Build history of the part. All positions in model axes, mm. Face numbers are marked on the shaded views. A direction names the side the tool comes from. Give positions to 0.01 mm unless a question says otherwise; leave off trailing zeros. Write each loop counter-clockwise with the first axis right and the second up, starting at its lowest first coordinate (ties: lowest second). Pieces come first, ordered by that corner, then holes. Notation, with made-up numbers: (50.5, -13) -> (104.5, -13) arc R11 ccw to (104.5, -5) -> close; hole circle Ø11 at (-16, -21). An arc over 180 degrees is marked (long way). Write item = value, one per line. Start each with the question number.
Q1. Saw through at A-A, the plane y = 0. List the corners of the cut face in (x, z).
Q2. Mould opens along Y. For the marked faces 4, 5 and 6 say: pulls with the +Y half, pulls with the -Y half, needs draft (parallel to the pull), parting line crosses it, or undercut.
Q3. Saw through at D-D, the plane y = -13.5. List the corners of the cut face in (x, z), then the cut area to 3 significant figures.
Q4. Tool access for the marked faces 1, 2 and 3: list every direction of +Z, -Z, +X, -X, +Y, -Y with a clear straight run to the whole face (end or side of a thin tool).
Q5. Drop flat-ended pins along their axis: P1, Ø4, axis at y = -4, z = 3.5, coming from the +X side; P2, Ø21, axis at x = 0, y = 0, coming from the +Z side; P3, Ø3, axis at x = 14.5, z = 3, coming from the +Y side. Give the stop position or say it passes through.
Q6. Wall check: line 1 (Y direction, x = 0, z = 3.5); line 2 (Y direction, x = 0, z = -0.5); line 3 (Z direction, x = -12, y = -19). Give the ranges that are in metal, low to high.
Q7. Saw through at C-C, the plane z = 4. List the corners of the cut face in (x, y), then the cut area to 3 significant figures.
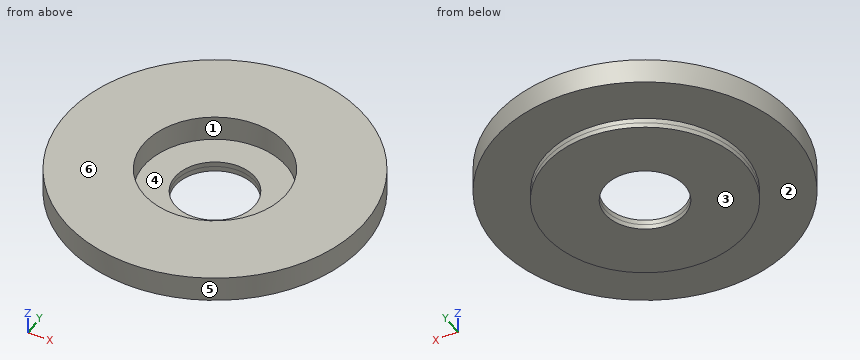
from build123d import *
from build123d.topology import SkipClean

# Parameters (mm, degrees)
SKETCH2_R           = 30
SKETCH2_R_2         = 8
BOSS_EXTRUDE1_DEPTH = 2
SKETCH3_R           = 30
SKETCH3_R_2         = 14.25
BOSS_EXTRUDE2_DEPTH = 5
CUT_EXTRUDE1_START  = -1
SKETCH5_R           = 14.25
SKETCH5_R_2         = 8
CUT_EXTRUDE1_DEPTH  = 1
SKETCH7_R           = 30
SKETCH7_R_2         = 14.25
BOSS_EXTRUDE4_DEPTH = 1
CUT_EXTRUDE3_START  = -2
SKETCH8_R           = 30
SKETCH8_R_2         = 14.25
CUT_EXTRUDE3_DEPTH  = 2
BOSS_EXTRUDE6_START = 1
SKETCH10_R          = 20
SKETCH10_R_2        = 8
BOSS_EXTRUDE6_DEPTH = 1
SKETCH11_R          = 30
SKETCH11_R_2        = 20
CUT_EXTRUDE4_DEPTH  = 1


with BuildPart() as part:
    # Sketch2 → Boss-Extrude1 (new body)
    with BuildSketch(Plane.XY):
        Circle(SKETCH2_R)
        Circle(SKETCH2_R_2, mode=Mode.SUBTRACT)
    extrude(amount=BOSS_EXTRUDE1_DEPTH)

    # Sketch3 → Boss-Extrude2 (add)
    with BuildSketch(Plane.XY.offset(2)):
        Circle(SKETCH3_R)
        Circle(SKETCH3_R_2, mode=Mode.SUBTRACT)
    extrude(amount=BOSS_EXTRUDE2_DEPTH)

    # Sketch5 → Cut-Extrude1 (cut)
    with BuildSketch(Plane.XY.offset(2).offset(CUT_EXTRUDE1_START)):
        Circle(SKETCH5_R)
        Circle(SKETCH5_R_2, mode=Mode.SUBTRACT)
    extrude(amount=CUT_EXTRUDE1_DEPTH, mode=Mode.SUBTRACT)

    # Sketch7 → Boss-Extrude4 (add)
    with BuildSketch(Plane.XY.offset(7)):
        Circle(SKETCH7_R)
        Circle(SKETCH7_R_2, mode=Mode.SUBTRACT)
    extrude(amount=BOSS_EXTRUDE4_DEPTH)

    # Sketch8 → Cut-Extrude3 (cut)
    with BuildSketch(Plane.XY.offset(8).offset(CUT_EXTRUDE3_START)):
        Circle(SKETCH8_R)
        Circle(SKETCH8_R_2, mode=Mode.SUBTRACT)
    extrude(amount=CUT_EXTRUDE3_DEPTH, mode=Mode.SUBTRACT)

    # Sketch10 → Boss-Extrude6 (add)
    with SkipClean():  # the faces are left unmerged after this step: merging them gives an invalid solid
        with BuildSketch(Plane(origin=(0, 0, 0), x_dir=(-1, 0, 0), z_dir=(0, 0, -1)).offset(BOSS_EXTRUDE6_START)):
            with Locations(Location((0, 0, 0), (0, 0, 180))):
                Circle(SKETCH10_R)
            Circle(SKETCH10_R_2, mode=Mode.SUBTRACT)
        extrude(amount=-BOSS_EXTRUDE6_DEPTH)

    # Sketch11 → Cut-Extrude4 (cut)
    with BuildSketch(Plane(origin=(0, 0, 0), x_dir=(-1, 0, 0), z_dir=(0, 0, -1))):
        Circle(SKETCH11_R)
        Circle(SKETCH11_R_2, mode=Mode.SUBTRACT)
    extrude(amount=-CUT_EXTRUDE4_DEPTH, mode=Mode.SUBTRACT)


solid = part.part
Report:
q1.outline = (-30, 1) -> (-20, 1) -> (-20, -1) -> (-8, -1) -> (-8, 1) -> (-14.25, 1) -> (-14.25, 6) -> (-30, 6) -> close; (8, -1) -> (20, -1) -> (20, 1) -> (30, 1) -> (30, 6) -> (14.25, 6) -> (14.25, 1) -> (8, 1) -> close
q2.face_4 = undercut
q2.face_5 = parting line crosses it
q2.face_6 = needs draft
q3.outline = (-26.79, 1) -> (-14.76, 1) -> (-14.76, -1) -> (14.76, -1) -> (14.76, 1) -> (26.79, 1) -> (26.79, 6) -> (4.56, 6) -> (4.56, 1) -> (-4.56, 1) -> (-4.56, 6) -> (-26.79, 6) -> close
q3.area = 281 mm2
q4.face_1 = +Z
q4.face_2 = -Z
q4.face_3 = -Z, +X, -X, +Y, -Y
q5.P1 = 29.93
q5.P2 = 1
q5.P3 = 27.04
q6.line_1 = -30 to -14.25, 14.25 to 30
q6.line_2 = -20 to -8, 8 to 20
q6.line_3 = 1 to 6
q7.outline = circle Ø60 at (0, 0); hole circle Ø28.5 at (0, 0)
q7.area = 2,190 mm2
